Check sheet for the modelled part. Datum: model origin and axes. Units: mm. Give positions to 0.01 mm unless a question says otherwise; leave off trailing zeros. Order: outer loops, then holes, each group sorted by start corner. A loop starts at its lowest first (then second) coordinate and runs counter-clockwise, first axis right, second up. Notation, with made-up numbers: M -26,17.25 L 6,17.25 A11 ccw 6,32.25 Z; hole C 57,-33 d3. An arc over 180 degrees is marked long. Answer in a Markdown table with one row per item. Add a question column.
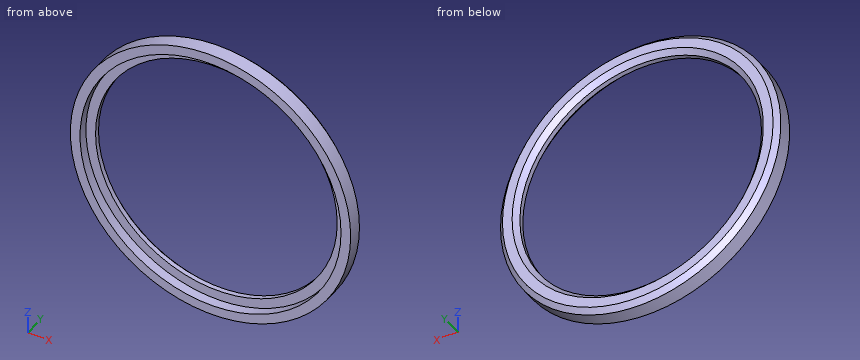
from build123d import *

# Parameters (mm, degrees)
SKETCH1_R           = 14.5
SKETCH1_R_2         = 12.5
BOSS_EXTRUDE1_DEPTH = 2
SKETCH2_R           = 13.5
CUT_EXTRUDE1_DEPTH  = 1
CHAMFER1_SIZE       = 0.5


with BuildPart() as part:
    # Sketch1 → Boss-Extrude1 (new body)
    with BuildSketch(Plane(origin=(0, 0, 0), x_dir=(1, 0, 0), z_dir=(0, 1, 0))):
        Circle(SKETCH1_R)
        Circle(SKETCH1_R_2, mode=Mode.SUBTRACT)
    extrude(amount=BOSS_EXTRUDE1_DEPTH)

    # Sketch2 → Cut-Extrude1 (cut)
    with BuildSketch(Plane.XZ):
        Circle(SKETCH2_R)
    extrude(amount=-CUT_EXTRUDE1_DEPTH, mode=Mode.SUBTRACT)

    # Chamfer1
    chamfer1_edges = [part.edges().sort_by_distance(p)[0] for p in [
        (-14.5, 2, 0),
        (-12.5, 2, 0),
    ]]
    chamfer(chamfer1_edges, length=CHAMFER1_SIZE)


solid = part.part
Q1. Cross-section at B-B (z = 0). Record the boundary of the cut face in (x, y).
Q2. Go/stop test with flat-tipped pins: pin 1 (15 mm diameter, centred on x = 0, z = 0, fed in from +Y); pin 2 (3 mm diameter, centred on x = -11.5, z = -10.5, fed in from +Y); pin 3 (1 mm diameter, centred on x = -7.5, y = 0.5, fed in from -Z). Record where each tip stops, or that it passes through.
Q3. Cross-section at A-A (x = 0). Record the boundary of the cut face in (y, z), and give its area (3 significant figures).
Q4. Thickness scan on probe 1 along Z at (x, y) = (0, 0.25); probe 2 along X at (y, z) = (1.25, 0); probe 3 along Y at (x, z) = (9.75, 9.25). Record the ranges inside material, lowest first.
Values follow:
| question | item | result |
|---|---|---|
| 1 | outline | M -14.5,0 L -13.5,0 L -13.5,1 L -12.5,1 L -12.5,1.5 L -13,2 L -14,2 L -14.5,1.5 Z; M 12.5,1 L 13.5,1 L 13.5,0 L 14.5,0 L 14.5,1.5 L 14,2 L 13,2 L 12.5,1.5 Z |
| 2 | pin 1 | through |
| 2 | pin 2 | y = 1.93 |
| 2 | pin 3 | z = -12.7 |
| 3 | outline | M 0,-14.5 L 1.5,-14.5 L 2,-14 L 2,-13 L 1.5,-12.5 L 1,-12.5 L 1,-13.5 L 0,-13.5 Z; M 0,13.5 L 1,13.5 L 1,12.5 L 1.5,12.5 L 2,13 L 2,14 L 1.5,14.5 L 0,14.5 Z |
| 3 | area | 5.50 mm² |
| 4 | probe 1 | -14.5 to -13.5, 13.5 to 14.5 |
| 4 | probe 2 | -14.5 to -12.5, 12.5 to 14.5 |
| 4 | probe 3 | 1 to 2 |
